Solid Edge part; units mm, degrees
sketch "Sketch1" plane through (0, 0, 0) normal (0, 0, 1) x (1, 0, 0)
  circle A0 centre (0, 0) radius 5
extrude "Protrusion1" add sketch "Sketch1" along normal blind 20
sketch "Sketch2" plane through (0, 0, 20) normal (0, 0, 1) x (1, 0, 0)
  circle A0 centre (0, 0) radius 4
extrude "ExtrudedProtrusion_2" add sketch "Sketch2" along normal blind 155
sketch "Sketch3" plane through (0, 0, 20) normal (0, 0, 1) x (0, -1, 0)
  line L0 (-3.8216, 6.2347) -> (3.8216, 6.2347)
  line L1 (3.8216, 6.2347) -> (3.8216, 4)
  line L2 (3.8216, 4) -> (0, 4)
  line L3 (0, 4) -> (-3.8216, 4)
  line L4 (-3.8216, 4) -> (-3.8216, 6.2347)
extrude "ExtrudedCutout_1" cut sketch "Sketch3" against normal blind 5
sketch "Sketch4" plane through (0, 0, 175) normal (0, 0, 1) x (0, -1, 0)
  line L0 (-3.2306, 4) -> (4.2507, 4)
  line L1 (4.2507, 4) -> (4.2507, 2.6458)
  line L2 (4.2507, 2.6458) -> (0, 2.6458)
  line L3 (0, 2.6458) -> (-3.2306, 2.6458)
  line L4 (-3.2306, 2.6458) -> (-3.2306, 4)
extrude "ExtrudedCutout_2" cut sketch "Sketch4" against normal blind 5
sketch "Sketch5" plane through (0, 0, 0) normal (0, 0, -1) x (-1, 0, 0)
  circle A0 centre (0, 0) radius 8.5
extrude "ExtrudedProtrusion_6" add sketch "Sketch5" along normal blind 5
sketch "Sketch6" plane through (0, 0, -5) normal (0, 0, -1) x (-1, 0, 0)
  circle A0 centre (0, 0) radius 7.5
extrude "ExtrudedProtrusion_7" add sketch "Sketch6" along normal blind 10
The listing builds one solid part. Answer for the finished solid, in the listing's coordinates (mm). A direction names the side the tool comes from. Give positions to 0.01 mm unless a question says otherwise; leave off trailing zeros. Write each loop counter-clockwise with the first axis right and the second up, starting at its lowest first coordinate (ties: lowest second). Pieces come first, ordered by that corner, then holes.
Item 1: Which of the six approach directions +Z, -Z, +X, -X, +Y, -Y give full straight-line access (tool end or side, diameter ignored) to faces 1 (the cylindrical face through (7.493, -0.33, -9.93)), 2 (the cylindrical face through (-0.867, 3.905, 96.415)), 3 (the flat face through (2.646, 0, 173)), 4 (the cylindrical face through (-4.57, -7.167, -2.465))?
Item 2: Section A-A, the plane x = 0 is taken. Write down the section's boundary in (y, z), plus the area to 4 significant figures.
Item 3: Flat-ended cylindrical pins translate along their axes: P1, Ø5, axis at x = -6, z = 122, coming from the -Y side; P2, Ø6, axis at x = 1, z = 83, coming from the -Y side; P3, Ø5, axis at x = 5, y = 3, coming from the +Z side; P4, Ø4, axis at y = -1, z = 17.5, coming from the +X side. Find the tip coordinate at first contact, or state that the pin passes through.
Item 4: Find the intervals of material crossed by line 1 along Y through (x, z) = (0.25, 163.5); line 2 along Z through (x, y) = (-4.5, -4.25); line 3 along Z through (x, y) = (7.5, 1.5), in increasing order.
Item 5: Section B-B, the plane z = 104.5 is taken. Write down the section's boundary in (x, y).
Completed:
1. face 1: -Z
1. face 2: +Z
1. face 3: +Z, +X, +Y, -Y
1. face 4: +Z, -Z
2. outline: (-8.5, -5) - (-7.5, -5) - (-7.5, -15) - (7.5, -15) - (7.5, -5) - (8.5, -5) - (8.5, 0) - (5, 0) - (5, 20) - (4, 20) - (4, 175) - (-4, 175) - (-4, 20) - (-5, 20) - (-5, 0) - (-8.5, 0) - close
2. area: 1,675 mm2
3. P1: stops at y = -1.94
3. P2: stops at y = -4
3. P3: stops at z = 175
3. P4: stops at x = 4
4. line 1: y = -3.99 to 3.99
4. line 2: z = -15 to 0
4. line 3: z = -5 to 0
5. outline: circle Ø8 at (0, 0)
